The listing builds one solid part. Answer for the finished solid, in the listing's coordinates (mm). A direction names the side the tool comes from. Coordinates: 2 decimals unless noted, no trailing zeros. Order: outer loops, then holes, each group sorted by start corner. A loop starts at its lowest first (then second) coordinate and runs counter-clockwise, first axis right, second up.
```python
from build123d import *

# Parameters (mm, degrees)
F0_R     = 5.5
F0_W     = 9.9
F0_H     = 3
F0_W_2   = 15
F0_H_2   = 3.05
F0_W_3   = 3.05
F0_H_3   = 15
F1_DEPTH = 3


with BuildPart() as f1:
    # F0 (on Right) → F1 (new body)
    with BuildSketch(Plane.YZ):
        Polygon((17, 7.5), (17, 16.5), (7.5, 16.5), (-7.5, 16.5), (-17, 16.5), (-17, 7.5), (-17, -7.5), (-17, -16.5), (-7.45, -16.5), (-7.45, -13.45), (7.45, -13.45), (7.45, -16.5), (17, -16.5), (17, -7.5), align=None)
        with Locations((0, -5.975)):
            Circle(F0_R, mode=Mode.SUBTRACT)
        with Locations((0, 5)):
            Rectangle(F0_W, F0_H, mode=Mode.SUBTRACT)
        with Locations((0, 18.025)):
            Rectangle(F0_W_2, F0_H_2)
        with Locations((-18.525, 0)):
            Rectangle(F0_W_3, F0_H_3)
        with Locations((18.525, 0)):
            Rectangle(F0_W_3, F0_H_3)
    extrude(amount=F1_DEPTH)


solid = f1.part
```
(1) Find section D-D (y = 10.5). Write down the section's boundary in (x, z).
(2) Find section B-B (y = -0.5). Write down the section's boundary in (x, z).
(3) Consider line 1 (Z direction, x = 1.75, y = 0) (3 decimals); line 2 (Y direction, x = 1.45, z = -6); line 3 (Y direction, x = 2.1, z = 14). Determine where each line is inside the solid, lowest interval first.
(4) Find section A-A (z = 6). Write down the section's boundary in (x, y).
(5) Find section C-C (x = 1.95). Write down the section's boundary in (y, z) (3 decimals).
(6) Each of these flat-tipped pins is pushed along its axis until it touches: pin 1 Ø1.5 at (x, y) = (1, 8.5) entering from +Z; pin 2 Ø0.9 at (x, z) = (1, 18.5) entering from +Y; pin 3 Ø1.5 at (x, z) = (2, 11.5) entering from +Y. Where does it stop, or does it pass through?
(7) For faces 4 (the face through (1, -4.95, 5)), 5 (the face through (1, 7.5, 18)), 6 (the face through (1, -12, 16.5)), 7 (the face through (1, 7.45, -15)), 8 (the face through (1, -17, -12)), determine the directions among +Z, -Z, +X, -X, +Y, -Y from which every point of the face is accessible in a straight line to the end or side of a thin tool.
(8) The mould has two halves that part along Y. Classify faces 1 (the face through (1, 19, 7.5)), 2 (the face through (1, 0, 3.5)), 3 (the face through (1, -17, 12)): released by +Y, released by -Y, zero draft, split by the parting line, or undercut.
Findings below:
1. outline: (0, -16.5) - (3, -16.5) - (3, 16.5) - (0, 16.5) - close
2. outline: (0, -13.45) - (3, -13.45) - (3, -11.45) - (0, -11.45) - close; (0, -0.5) - (3, -0.5) - (3, 3.5) - (0, 3.5) - close; (0, 6.5) - (3, 6.5) - (3, 19.55) - (0, 19.55) - close
3. line 1: z = -13.45 to -11.475, -0.475 to 3.5, 6.5 to 19.55
3. line 2: y = -20.05 to -5.5, 5.5 to 20.05
3. line 3: y = -17 to 17
4. outline: (0, -20.05) - (3, -20.05) - (3, -4.95) - (0, -4.95) - close; (0, 4.95) - (3, 4.95) - (3, 20.05) - (0, 20.05) - close
5. outline: (-20.05, -7.5) - (-17, -7.5) - (-17, -16.5) - (-7.45, -16.5) - (-7.45, -13.45) - (7.45, -13.45) - (7.45, -16.5) - (17, -16.5) - (17, -7.5) - (20.05, -7.5) - (20.05, 7.5) - (17, 7.5) - (17, 16.5) - (7.5, 16.5) - (7.5, 19.55) - (-7.5, 19.55) - (-7.5, 16.5) - (-17, 16.5) - (-17, 7.5) - (-20.05, 7.5) - close; hole circle Ø11 at (0, -5.975); hole (-4.95, 3.5) - (4.95, 3.5) - (4.95, 6.5) - (-4.95, 6.5) - close
6. pin 1: stops at z = 16.5
6. pin 2: stops at y = 7.5
6. pin 3: stops at y = 17
7. face 4: +X, -X
7. face 5: +Z, +X, -X, +Y
7. face 6: +Z, +X, -X, -Y
7. face 7: -Z, +X, -X
7. face 8: -Z, +X, -X, -Y
8. face 1: zero draft
8. face 2: undercut
8. face 3: released by -Y
